from build123d import *

# Parameters (mm, degrees)
SKETCH1_W                = 406.4
SKETCH1_H                = 457.2
BOSS_EXTRUDE1_DEPTH      = 5.715
SKETCH4_W                = 25.4
SKETCH4_H                = 5.715
FRONT_JIGSAW_DEPTH       = 6.715
SKETCH5_W                = 5.715
SKETCH5_H                = 25.4
RIGHT_JIGSAW_DEPTH       = 6.715
SKETCH7_W                = 5.715
SKETCH7_H                = 12.7
CENTER_SUPPORT_JIG_DEPTH = 6.715


with BuildPart() as part:
    # Sketch1 → Boss-Extrude1 (new body)
    with BuildSketch(Plane.XY):
        Rectangle(SKETCH1_W, SKETCH1_H)
    extrude(amount=BOSS_EXTRUDE1_DEPTH)

    # Sketch4 → Front Jigsaw (cut, through all)
    with BuildSketch(Plane(origin=(0, 0, 0), x_dir=(-1, 0, 0), z_dir=(0, 0, -1))):
        with Locations((-114.3, -225.7425)):
            Rectangle(SKETCH4_W, SKETCH4_H)
        with Locations((-190.5, -225.7425)):
            Rectangle(SKETCH4_W, SKETCH4_H)
        with Locations((-38.1, -225.7425)):
            Rectangle(SKETCH4_W, SKETCH4_H)
        with Locations((38.1, -225.7425)):
            Rectangle(SKETCH4_W, SKETCH4_H)
        with Locations((114.3, -225.7425)):
            Rectangle(SKETCH4_W, SKETCH4_H)
        with Locations((190.5, -225.7425)):
            Rectangle(SKETCH4_W, SKETCH4_H)
    front_jigsaw = extrude(amount=-FRONT_JIGSAW_DEPTH, mode=Mode.SUBTRACT)

    # Back Jigsaw: Front Jigsaw across plane
    add(front_jigsaw.mirror(Plane.ZX), mode=Mode.SUBTRACT)

    # Sketch5 → Right Jigsaw (cut, through all)
    with BuildSketch(Plane(origin=(0, 0, 0), x_dir=(-1, 0, 0), z_dir=(0, 0, -1))):
        with Locations((200.3425, 190.5)):
            Rectangle(SKETCH5_W, SKETCH5_H)
        with Locations((200.3425, 114.3)):
            Rectangle(SKETCH5_W, SKETCH5_H)
        with Locations((200.3425, 38.1)):
            Rectangle(SKETCH5_W, SKETCH5_H)
        with Locations((200.3425, -38.1)):
            Rectangle(SKETCH5_W, SKETCH5_H)
        with Locations((200.3425, -114.3)):
            Rectangle(SKETCH5_W, SKETCH5_H)
        with Locations((200.3425, -190.5)):
            Rectangle(SKETCH5_W, SKETCH5_H)
    right_jigsaw = extrude(amount=-RIGHT_JIGSAW_DEPTH, mode=Mode.SUBTRACT)

    # Left Jigsaw: Right Jigsaw across plane
    add(right_jigsaw.mirror(Plane(origin=(0, 0, 0), x_dir=(0, 0, 1), z_dir=(1, 0, 0))), mode=Mode.SUBTRACT)

    # Sketch7 → Center Support Jig (cut, through all)
    with BuildSketch(Plane(origin=(0, 0, 0), x_dir=(-1, 0, 0), z_dir=(0, 0, -1))):
        with Locations((0, 12.7)):
            Rectangle(SKETCH7_W, SKETCH7_H)
        with Locations((0, -12.7)):
            Rectangle(SKETCH7_W, SKETCH7_H)
    extrude(amount=-CENTER_SUPPORT_JIG_DEPTH, mode=Mode.SUBTRACT)


solid = part.part
Geometry: final body of the model. Coordinates: model frame, mm. Give positions to 0.01 mm unless a question says otherwise; leave off trailing zeros. Write each loop counter-clockwise with the first axis right and the second up, starting at its lowest first coordinate (ties: lowest second). Pieces come first, ordered by that corner, then holes. Notation, with made-up numbers: M 46.5,61.5 L 94.5,61.5 A7 cw 94.5,72.5 Z; hole C -18.5,53.25 d8. An arc over 180 degrees is marked long. Answer in a Markdown table with one row per item. Add a question column.
(1) Section B-B on z = 3.9. State how many separate pieces and enclosed holes the cut face has, and give its area (3 significant figures).
(2) Section A-A on y = -112.5. Return loops of the section in (x, z) (3 decimals), and give its area (3 significant figures).
(3) Ray query, line 1 (Y direction, x = 0, z = 1.6); line 2 (X direction, y = -15, z = 2); line 3 (X direction, y = 102.5, z = 1.2) (3 decimals). Return the intervals inside material, ascending.
(4) First-contact query: pin 1 (2 mm diameter, centred on x = 123.5, z = 1.5, fed in from -Y) (3 decimals); pin 2 (3 mm diameter, centred on x = -199.5, z = 2.5, fed in from +Y) (3 decimals); pin 3 (3 mm diameter, centred on y = 224.5, z = 1.5, fed in from -X). Flat tips, straight axial feed; report the tip coordinate or a pass-through.
Result set:
| question | item | result |
|---|---|---|
| 1 | separate pieces | 1 |
| 1 | enclosed holes | 2 |
| 1 | area | 182,000 mm^2 |
| 2 | outline | M -197.485,0 L 197.485,0 L 197.485,5.715 L -197.485,5.715 Z |
| 2 | area | 2,260 mm^2 |
| 3 | line 1 | y = -228.6 to -19.05, -6.35 to 6.35, 19.05 to 228.6 |
| 3 | line 2 | x = -203.2 to -2.86, 2.86 to 203.2 |
| 3 | line 3 | x = -197.485 to 197.485 |
| 4 | pin 1 | stops at y = -222.885 |
| 4 | pin 2 | stops at y = 222.885 |
| 4 | pin 3 | stops at x = -177.8 |
